```python
from build123d import *

# Parameters (mm, degrees)
SKETCH2_R          = 40
SKETCH2_R_2        = 32
CUT_EXTRUDE1_DEPTH = 10
FILLET1_R          = 5
CHAMFER1_SIZE      = 5


with BuildPart() as part:
    # Sketch1 → Revolve1 (revolve)
    with BuildSketch(Plane.XY):
        with BuildLine():
            Line((40, -57.445626465), (40, -282.445626465))
            Line((40, -282.445626465), (0, -282.445626465))
            Line((0, -282.445626465), (0, 70))
            ThreePointArc((0, 70), (66.787700412, 20.961943462), (40, -57.445626465))
        make_face()
    revolve(axis=Axis((0, 0, 0), (0, -1, 0)))

    # Sketch2 → Cut-Extrude1 (cut)
    with BuildSketch(Plane(origin=(0, -162.445626465, 0), x_dir=(-1, 0, 0), z_dir=(0, -1, 0))):
        with Locations(Location((0, 0, 0), (0, 0, 270))):
            Circle(SKETCH2_R)
        with Locations(Location((0, 0, 0), (0, 0, 90))):
            Circle(SKETCH2_R_2, mode=Mode.SUBTRACT)
    extrude(amount=-CUT_EXTRUDE1_DEPTH, mode=Mode.SUBTRACT)

    # Fillet1
    fillet1_edges = [part.edges().sort_by_distance(p)[0] for p in [
        (-40, -57.445626465, 0),
    ]]
    fillet(fillet1_edges, radius=FILLET1_R)

    # Chamfer1
    chamfer1_edges = [part.edges().sort_by_distance(p)[0] for p in [
        (-40, -152.445626465, 0),
        (-40, -162.445626465, 0),
        (-40, -282.445626465, 0),
    ]]
    chamfer(chamfer1_edges, length=CHAMFER1_SIZE)


solid = part.part
```
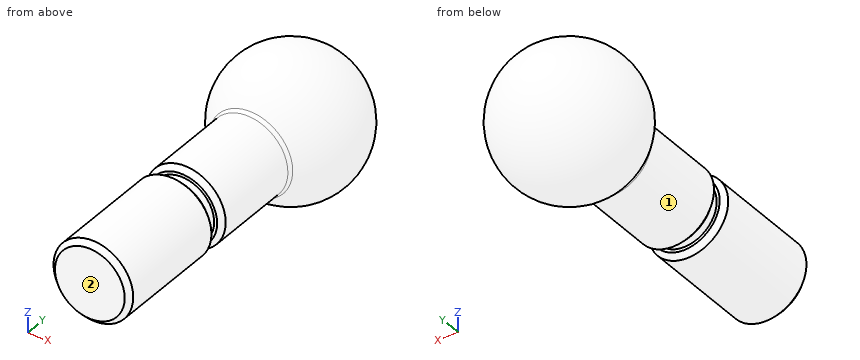
Input: part model. Units: mm. Frame: model coordinates. Face numbers are marked on the shaded views. A direction names the side the tool comes from. Give positions to 0.01 mm unless a question says otherwise; leave off trailing zeros. Write each loop counter-clockwise with the first axis right and the second up, starting at its lowest first coordinate (ties: lowest second). Pieces come first, ordered by that corner, then holes. Notation, with made-up numbers: (69.25, 52.25) - (128.25, 52.25) arc R28 cw to (128.25, 90.25) - close; hole circle Ø1 at (49, 49.25). An arc over 180 degrees is marked (long way). Write item = value, one per line. Start each with the question number.
1) Material intervals for L1, parallel to Z at x = 1, y = -128; L2, parallel to Z at x = -25, y = -135.5; L3, parallel to X at y = 44, z = -49.5, sorted ascending. Write a range as [from, to].
2) Reachability of the marked faces 1 and 2 from +Z, -Z, +X, -X, +Y, -Y: full face, straight path, thin tool, end or side. Return the list, or none.
3) Cut plane A-A (y = -196). Return loops of the section in (x, z).
4) Pin query (flat end, axial travel): pin 1 (4 mm diameter, centred on y = -23, z = 36.5, fed in from +X); pin 2 (8 mm diameter, centred on x = 20.5, y = -69.5, fed in from -Z); pin 3 (4 mm diameter, centred on x = -5.5, z = -49, fed in from -Y). Return the tip coordinate at first contact, or that it passes through.
5) Cut plane B-B (z = -57). Return loops of the section in (x, y) (1 decimal), and give its area (3 significant figures).
Answers follow:
q1.L1 = [-39.99, 39.99]
q1.L2 = [-31.22, 31.22]
q1.L3 = [-22.67, 22.67]
q2.face_1 = -Y
q2.face_2 = +Z, -Z, +X, -X, -Y
q3.outline = circle Ø80 at (0, 0)
q4.pin_1 = 56.63
q4.pin_2 = -36.44
q4.pin_3 = -51.59
q5.outline = circle Ø81.3 at (0, 0)
q5.area = 5,190 mm^2
